The model under review builds one solid part; all positions refer to its coordinate system, in mm. A direction names the side the tool comes from. Give positions to 0.01 mm unless a question says otherwise; leave off trailing zeros. Write each loop counter-clockwise with the first axis right and the second up, starting at its lowest first coordinate (ties: lowest second). Pieces come first, ordered by that corner, then holes. Notation, with made-up numbers: (53.5, -22) -> (60.5, -22) arc R34 cw to (60.5, 15) -> close; hole circle Ø10 at (89.25, 37.5). An arc over 180 degrees is marked (long way). Use CSV: the item, a comma, the result in double quotes.
```python
from build123d import *

# Parameters (mm, degrees)
F1_DEPTH      = 6
F2_R          = 1
F3_DEPTH      = 25
F5_DEPTH      = 6
F6_DEPTH      = 10
F11_R         = 1
F12_T1_DEPTH  = 5
F12_T3_DEPTH  = 11
F12_T8_ANGLE  = 359.64
F12_T14_ANGLE = 359.64
F12_T21_DEPTH = 12.5
F12_T25_DEPTH = 18.5
F12_T32_DEPTH = 18.5
F12_T36_DEPTH = 12.5
F13_R         = 1.5
F14_DEPTH     = 25


# Not quite as in the source:
# - a fillet or chamfer that OpenCascade refuses, or shapes differently, is made with other operations: its cross-section is extruded or revolved along the edge and cut away or added


with BuildPart() as f1:
    # F0 (on Front) → F1 (new body)
    with BuildSketch(Plane.XZ):
        with BuildLine():
            Line((2.5, -7.3357003756), (2.5, -18.4552618332))
            Line((2.5, -18.4552618332), (5.5, -18.4552618332))
            Line((5.5, -18.4552618332), (5.5, -9.236476601))
            ThreePointArc((5.5, -9.236476601), (10.75, 0), (5.5, 9.236476601))
            Line((5.5, 9.236476601), (5.5, 14.236476601))
            Line((5.5, 14.236476601), (2.5, 14.236476601))
            Line((2.5, 14.236476601), (2.5, 7.3357003756))
            ThreePointArc((2.5, 7.3357003756), (7.75, 0), (2.5, -7.3357003756))
        make_face()
    extrude(amount=F1_DEPTH)


with BuildPart() as f1b:
    # F0 (on Front) → F1, piece 2 (new body)
    with BuildSketch(Plane.XZ):
        with BuildLine():
            ThreePointArc((-2.5, -7.3357003756), (-7.75, 0), (-2.5, 7.3357003756))
            Line((-2.5, 7.3357003756), (-2.5, 14.236476601))
            Line((-2.5, 14.236476601), (-5.5, 14.236476601))
            Line((-5.5, 14.236476601), (-5.5, 9.236476601))
            ThreePointArc((-5.5, 9.236476601), (-10.75, 0), (-5.5, -9.236476601))
            Line((-5.5, -9.236476601), (-5.5, -18.4552618332))
            Line((-5.5, -18.4552618332), (-2.5, -18.4552618332))
            Line((-2.5, -18.4552618332), (-2.5, -7.3357003756))
        make_face()
    extrude(amount=F1_DEPTH)


with BuildPart() as f3_tool:
    # F2 (on face) → F3 (new body)
    with BuildSketch(Plane.YZ.offset(5.5)):
        with Locations((-3, 11.7896459997)):
            Circle(F2_R)
    extrude(amount=-F3_DEPTH)


with BuildPart() as f1_1:
    add(f1.part)

    # F3: cut by f3_tool
    add(f3_tool.part, mode=Mode.SUBTRACT)


with BuildPart() as f1b_1:
    add(f1b.part)

    # F3: cut by f3_tool
    add(f3_tool.part, mode=Mode.SUBTRACT)


with BuildPart() as f5:
    # F4 (on Front) → F5 (new body)
    with BuildSketch(Plane.XZ):
        Polygon((2.5, -12.8954811044), (-2.5, -12.8954811044), (-2.5, -18.4552618332), (-2.5, -20.8968445659), (2.5, -20.8968445659), (2.5, -18.4552618332), align=None)
    extrude(amount=F5_DEPTH)


with BuildPart() as f6:
    # F4 (on Front) → F6 (new body, symmetric)
    with BuildSketch(Plane.XZ):
        Polygon((2.5, -20.8968445659), (-2.5, -20.8968445659), (-15, -20.8968445659), (-15, -23.8968445659), (15, -23.8968445659), (15, -20.8968445659), align=None)
    extrude(amount=F6_DEPTH, both=True)


with BuildPart() as f6_1:
    # F7: moved
    add(f6.part.moved(Location((0, 0, 2.5))))


with BuildPart() as f5_1:
    # F7: moved
    add(f5.part.moved(Location((0, 0, 2.5))))


with BuildPart() as f6_2:
    # F8: moved
    add(f6_1.part.moved(Location((0, 4, 0))))


with BuildPart() as f5_2:
    add(f5_1.part)

    # F9: union F6
    add(f6_2.part)

    # F10: union F1, F1b
    add(f1_1.part)
    add(f1b_1.part)

    # F11
    f11_edges = [f5_2.edges().sort_by_distance(p)[0] for p in [
        (-10.25, -6, -18.396845),
        (10.25, -6, -18.396845),
        (15, 4, -18.396845),
        (0, 14, -18.396845),
        (-15, 4, -18.396845),
    ]]
    fillet(f11_edges, radius=F11_R)

    # F12: fillet of radius 3 on 7 edges, made by hand

    # F12_s2 → F12_t1 (join)
    with BuildSketch(Plane.XZ):
        with BuildLine():
            ThreePointArc((-8.5, -18.3968445659), (-6.3786796564, -17.5181649094), (-5.5, -15.3968445659))
            Line((-5.5, -15.3968445659), (-5.5, -18.3968445659))
            Line((-5.5, -18.3968445659), (-8.5, -18.3968445659))
        make_face()
        with BuildLine():
            ThreePointArc((8.5, -18.3968445659), (6.3786796564, -17.5181649094), (5.5, -15.3968445659))
            Line((5.5, -15.3968445659), (5.5, -18.3968445659))
            Line((5.5, -18.3968445659), (8.5, -18.3968445659))
        make_face()
    extrude(amount=F12_T1_DEPTH)

    # F12_s4 → F12_t3 (join)
    with BuildSketch(Plane.YZ.offset(-5.5)):
        with BuildLine():
            ThreePointArc((3, -18.3968445659), (0.8786796564, -17.5181649094), (0, -15.3968445659))
            Line((0, -15.3968445659), (0, -18.3968445659))
            Line((0, -18.3968445659), (3, -18.3968445659))
        make_face()
    extrude(amount=F12_T3_DEPTH)


with BuildPart() as f12_tool6:
    # F12_s7 → F12_t8 (revolve)
    with BuildSketch(Plane.XZ.offset(5)):
        with BuildLine():
            ThreePointArc((-8.5, -18.3968445659), (-6.3786796564, -17.5181649094), (-5.5, -15.3968445659))
            Line((-5.5, -15.3968445659), (-5.5, -18.3968445659))
            Line((-5.5, -18.3968445659), (-8.5, -18.3968445659))
        make_face()
    revolve(axis=Axis((-5.5, -5, -19.3968445659), (1, 0, 0)), revolution_arc=F12_T8_ANGLE)

    split(bisect_by=Plane.XZ.offset(6), keep=Keep.BOTTOM)

    split(bisect_by=Plane.XY.offset(-21.3968445659), keep=Keep.TOP)


with BuildPart() as f5_3:
    add(f5_2.part)

    # F12_t5: union F12_tool6
    add(f12_tool6.part)


with BuildPart() as f12_tool12:
    # F12_s13 → F12_t14 (revolve)
    with BuildSketch(Plane.XZ.offset(5)):
        with BuildLine():
            ThreePointArc((8.5, -18.3968445659), (6.3786796564, -17.5181649094), (5.5, -15.3968445659))
            Line((5.5, -15.3968445659), (5.5, -18.3968445659))
            Line((5.5, -18.3968445659), (8.5, -18.3968445659))
        make_face()
    revolve(axis=Axis((5.5, -5, -19.3968445659), (1, 0, 0)), revolution_arc=F12_T14_ANGLE)

    split(bisect_by=Plane.XZ.offset(6), keep=Keep.BOTTOM)

    split(bisect_by=Plane.XY.offset(-21.3968445659), keep=Keep.TOP)


with BuildPart() as f5_4:
    add(f5_3.part)

    # F12_t11: union F12_tool12
    add(f12_tool12.part)


with BuildPart() as f12_tool19:
    # F12_s20 → F12_t21 (new body)
    with BuildSketch(Plane.XZ.offset(5)):
        with BuildLine():
            ThreePointArc((-8.5, -18.3968445659), (-6.3786796564, -17.5181649094), (-5.5, -15.3968445659))
            Line((-5.5, -15.3968445659), (-5.5, -18.3968445659))
            Line((-5.5, -18.3968445659), (-8.5, -18.3968445659))
        make_face()
    extrude(amount=-F12_T21_DEPTH)

    split(bisect_by=Plane.XZ, keep=Keep.BOTTOM)


with BuildPart() as f12_tool23:
    # F12_s24 → F12_t25 (new body)
    with BuildSketch(Plane.YZ.offset(-13)):
        with BuildLine():
            ThreePointArc((3, -18.3968445659), (0.8786796564, -17.5181649094), (0, -15.3968445659))
            Line((0, -15.3968445659), (0, -18.3968445659))
            Line((0, -18.3968445659), (3, -18.3968445659))
        make_face()
    extrude(amount=F12_T25_DEPTH)

    split(bisect_by=Plane.YZ.offset(-5.5), keep=Keep.BOTTOM)


with BuildPart() as f12_tool19_1:
    add(f12_tool19.part)

    # F12_t27: intersect F12_tool23
    add(f12_tool23.part, mode=Mode.INTERSECT)


with BuildPart() as f5_5:
    add(f5_4.part)

    # F12_t17: union F12_tool19
    add(f12_tool19_1.part)


with BuildPart() as f12_tool30:
    # F12_s31 → F12_t32 (new body)
    with BuildSketch(Plane.YZ.offset(-5.5)):
        with BuildLine():
            ThreePointArc((3, -18.3968445659), (0.8786796564, -17.5181649094), (0, -15.3968445659))
            Line((0, -15.3968445659), (0, -18.3968445659))
            Line((0, -18.3968445659), (3, -18.3968445659))
        make_face()
    extrude(amount=F12_T32_DEPTH)

    split(bisect_by=Plane.YZ.offset(5.5), keep=Keep.TOP)


with BuildPart() as f12_tool34:
    # F12_s35 → F12_t36 (new body)
    with BuildSketch(Plane.XZ.offset(-7.5)):
        with BuildLine():
            ThreePointArc((8.5, -18.3968445659), (6.3786796564, -17.5181649094), (5.5, -15.3968445659))
            Line((5.5, -15.3968445659), (5.5, -18.3968445659))
            Line((5.5, -18.3968445659), (8.5, -18.3968445659))
        make_face()
    extrude(amount=F12_T36_DEPTH)

    split(bisect_by=Plane.XZ, keep=Keep.BOTTOM)


with BuildPart() as f12_tool30_1:
    add(f12_tool30.part)

    # F12_t38: intersect F12_tool34
    add(f12_tool34.part, mode=Mode.INTERSECT)


with BuildPart() as f5_6:
    add(f5_5.part)

    # F12_t28: union F12_tool30
    add(f12_tool30_1.part)

    # F13 (on face) → F14 (cut)
    with BuildSketch(Plane.XY.offset(-18.3968445659)):
        with Locations((-10, 9)):
            Circle(F13_R)
        with Locations((10, 9)):
            Circle(F13_R)
    extrude(amount=-F14_DEPTH, mode=Mode.SUBTRACT)


solid = f5_6.part
```
Q1. Consider section D-D (x = -10). Write out the cut boundary in (y, z), then the cut area to 3 significant figures.
Derived:
outline,"(-6, -21.4) -> (7.5, -21.4) -> (7.5, -18.4) -> (-5, -18.4) arc R1 ccw to (-6, -19.4) -> close; (-6, -3.94) -> (0, -3.94) -> (0, 3.94) -> (-6, 3.94) -> close; (10.5, -21.4) -> (14, -21.4) -> (14, -19.4) arc R1 ccw to (13, -18.4) -> (10.5, -18.4) -> close"
area,"97.9 mm2"
Q2. Machinability: for faces 4 (the flat face through (0, -3, -10.395)), 5 (the cylindrical face through (11.704, -5.715, -18.698)), 6 (the flat face through (5.5, -3, -12)), 7 (the flat face through (-5.5, -3, 13)), 8 (the cylindrical face through (-7.75, -2.96, -0.13)), which of the approach directions +Z, -Z, +X, -X, +Y, -Y give a long, thin tool a straight path to every point of the face, cutting with its end or side? Answer none if there is none.
Derived:
face 4,"+Z, +Y, -Y"
face 5,"+X, -Y"
face 6,"+X, +Y, -Y"
face 7,"+Z, -X, +Y, -Y"
face 8,"+Y, -Y"
Q3. Consider section C-C (z = -5.5). Write out the cut boundary in (x, y).
Derived:
outline,"(-9.24, -6) -> (-5.46, -6) -> (-5.46, 0) -> (-9.24, 0) -> close; (5.46, -6) -> (9.24, -6) -> (9.24, 0) -> (5.46, 0) -> close"
Q4. Consider section B-B (x = -3.5). Write out the cut boundary in (y, z), then the cut area to 3 significant figures.
Derived:
outline,"(-6, -21.4) -> (14, -21.4) -> (14, -19.4) arc R1 ccw to (13, -18.4) -> (3, -18.4) arc R3 cw to (0, -15.4) -> (0, -6.91) -> (-6, -6.91) -> close; (-6, 6.91) -> (0, 6.91) -> (0, 14.24) -> (-6, 14.24) -> close; hole circle Ø2 at (-3, 11.79)"
area,"171 mm2"
Q5. To check wall thickness, follow probe 1 along X at (y, z) = (-2, 12.5); probe 2 along Z at (x, y) = (3.85, -3); probe 3 along X at (y, z) = (-3, -14.5). State the ranges of each line that lie inside material, in increasing order.
Derived:
probe 1,"x = -5.5 to -2.5, 2.5 to 5.5"
probe 2,"z = -21.4 to -6.73, 6.73 to 10.79, 12.79 to 14.24"
probe 3,"x = -5.5 to 5.5"
Q6. The part is to be moulded in two halves that separate along Y. For faces 1 (the flat face through (5, 0, -7)), 2 (the flat face through (5.5, -3, 13)), 3 (the cylindrical face through (4.02, -3.13, 12.78)), say which applies: pulls with the +Y half, pulls with the -Y half, needs draft (parallel to the pull), parting line crosses it, or undercut.
Derived:
face 1,"pulls with the +Y half"
face 2,"needs draft"
face 3,"undercut"
Q7. Insertion check: pin 1 (1.5 mm diameter, centred on x = -1.5, z = -11.5, fed in from +Y); pin 2 (1.8 mm diameter, centred on y = -3.5, z = 10.5, fed in from -X); pin 3 (10 mm diameter, centred on x = 3.5, y = 8, fed in from +Z). Each pin has a flat end and moves straight along its axis. Give the tip position at first contact, or say it passes through.
Derived:
pin 1,"stops at y = 0"
pin 2,"stops at x = -5.5"
pin 3,"stops at z = -18.4"
Q8. Consider section A-A (y = -3). State how many separate pieces and enclosed holes the cut face has, then the cut area to 3 significant figures.
Derived:
separate pieces,"3"
enclosed holes,"0"
area,"342 mm2"
